```python
from build123d import *

# Parameters (mm, degrees)
SKETCH1_W           = 30
SKETCH1_H           = 60
SKETCH1_R           = 2
BOSS_EXTRUDE1_DEPTH = 3
SKETCH2_W           = 24
SKETCH2_H           = 3
BOSS_EXTRUDE2_DEPTH = 15
SKETCH3_R           = 2
CUT_EXTRUDE1_DEPTH  = 65.830548355
BOSS_EXTRUDE3_DEPTH = 2
SKETCH4_R           = 2.8
CUT_EXTRUDE2_DEPTH  = 2


with BuildPart() as part:
    # Sketch1 → Boss-Extrude1 (new body)
    with BuildSketch(Plane.XY):
        Rectangle(SKETCH1_W, SKETCH1_H)
        with Locations((8, 20)):
            Circle(SKETCH1_R, mode=Mode.SUBTRACT)
        with Locations(Location((8, -20, 0), (0, 0, 180))):
            Circle(SKETCH1_R, mode=Mode.SUBTRACT)
        with Locations(Location((-8, 20, 0), (0, 0, 180))):
            Circle(SKETCH1_R, mode=Mode.SUBTRACT)
        with Locations((-8, -20)):
            Circle(SKETCH1_R, mode=Mode.SUBTRACT)
    extrude(amount=BOSS_EXTRUDE1_DEPTH)

    # Sketch2 → Boss-Extrude2 (add, symmetric)
    with BuildSketch(Plane(origin=(0, 0, 0), x_dir=(0, 0, -1), z_dir=(1, 0, 0))):
        with Locations((-15, -28.5)):
            Rectangle(SKETCH2_W, SKETCH2_H)
    extrude(amount=BOSS_EXTRUDE2_DEPTH, both=True)

    # Sketch3 → Cut-Extrude1 (cut, through all)
    with BuildSketch(Plane(origin=(0, -27, 0), x_dir=(1, 0, 0), z_dir=(0, 1, 0))):
        with Locations(Location((-8, -6, 0), (0, 0, 270))):
            Circle(SKETCH3_R)
        with Locations(Location((8, -6, 0), (0, 0, 270))):
            Circle(SKETCH3_R)
        with Locations(Location((-8, -21, 0), (0, 0, 270))):
            Circle(SKETCH3_R)
        with Locations(Location((8, -21, 0), (0, 0, 270))):
            Circle(SKETCH3_R)
    extrude(amount=-CUT_EXTRUDE1_DEPTH, mode=Mode.SUBTRACT)

    # Sketch6 → Boss-Extrude3 (add, symmetric)
    with BuildSketch(Plane(origin=(0, 0, 0), x_dir=(0, 0, -1), z_dir=(1, 0, 0))):
        Polygon((-3, 30), (-27, -27), (-3, -27), align=None)
    extrude(amount=BOSS_EXTRUDE3_DEPTH, both=True)

    # Sketch4 → Cut-Extrude2 (cut)
    with BuildSketch(Plane(origin=(0, -27, 0), x_dir=(1, 0, 0), z_dir=(0, 1, 0))):
        with Locations(Location((-8, -6, 0), (0, 0, 270))):
            Circle(SKETCH4_R)
        with Locations(Location((8, -6, 0), (0, 0, 270))):
            Circle(SKETCH4_R)
    extrude(amount=-CUT_EXTRUDE2_DEPTH, mode=Mode.SUBTRACT)


solid = part.part
```
Part model, mm, in its own coordinate system. A direction names the side the tool comes from. Round coordinates to 2 decimals unless told otherwise and drop trailing zeros. Order: outer loops, then holes, each group sorted by start corner. A loop starts at its lowest first (then second) coordinate and runs counter-clockwise, first axis right, second up. Notation, with made-up numbers: M 33,18.25 L 72,18.25 A25 cw 72,42.25 Z; hole C -5,9 d2. An arc over 180 degrees is marked long. Put each result on its own line as item: value. Start each with the question number.
1. Drill centre lines: probe 1 along Y at (x, z) = (-8, 1.35); probe 2 along X at (y, z) = (-27.35, 6); probe 3 along Z at (x, y) = (-7.5, -9.5). Where is each one in solid material? Low to high. Write a range as [from, to].
2. Tool access for faces 5 (the face through (-6, -29, 5)), 6 (the face through (-8, -27, 15)), 7 (the face through (9, -27, 15)): list every direction of +Z, -Z, +X, -X, +Y, -Y with a clear straight run to the whole face (end or side of a thin tool).
3. Two-plate mould, pull along Z, no slides. Class faces 1 (the face through (2, -11, 10)), 2 (the face through (5.267, -27.986, 5.393)), 3 (the face through (0, 0, 0)), 4 (the face through (9.352, -28.479, 19.526)): +Z half, -Z half, draft (parallel to the pull), parting line (faces both ways), or undercut.
4. Drop flat-ended pins along their axis: pin 1 (6.5 mm diameter, centred on x = 7.5, y = 12, fed in from +Z); pin 2 (8 mm diameter, centred on y = -0.5, z = 19, fed in from -X); pin 3 (4 mm diameter, centred on x = 5.5, z = 13, fed in from +Y); pin 4 (3 mm diameter, centred on x = -8, z = 6, fed in from -Y). Give the stop position or say it passes through.
5. Slice it at C-C on y = -20. List the corners of the cut face in (x, z).
6. Slice it at A-A on x = -8. List the corners of the cut face in (y, z).
7. Slice it at B-B on z = 5.5. List the corners of the cut face in (x, y) (1 decimal), then the cut area to 3 significant figures.
8. Slice it at D-D on x = -12.75. List the corners of the cut face in (y, z), then the cut area to 3 significant figures.
Findings:
1. probe 1: [-30, -22], [-18, 18], [22, 30]
1. probe 2: [-15, -10.8], [-5.2, 5.2], [10.8, 15]
1. probe 3: [0, 3]
2. face 5: +Y
2. face 6: +Z, -X, +Y
2. face 7: +Z, +X, +Y
3. face 1: draft
3. face 2: undercut
3. face 3: -Z half
3. face 4: undercut
4. pin 1: z = 3
4. pin 2: x = -2
4. pin 3: y = -27
4. pin 4: through
5. outline: M -15,0 L -10,0 L -10,3 L -15,3 Z; M -6,0 L 6,0 L 6,3 L 2,3 L 2,24.05 L -2,24.05 L -2,3 L -6,3 Z; M 10,0 L 15,0 L 15,3 L 10,3 Z
6. outline: M -30,0 L -22,0 L -22,3 L -27,3 L -27,3.2 L -29,3.2 L -29,4 L -30,4 Z; M -30,8 L -29,8 L -29,8.8 L -27,8.8 L -27,19 L -30,19 Z; M -30,23 L -27,23 L -27,27 L -30,27 Z; M -18,0 L 18,0 L 18,3 L -18,3 Z; M 22,0 L 30,0 L 30,3 L 22,3 Z
7. outline: M -15,-30 L -9.9,-30 L -9.9,-29 L -10.8,-29 L -10.8,-27 L -15,-27 Z; M -6.1,-30 L 6.1,-30 L 6.1,-29 L 5.2,-29 L 5.2,-27 L 2,-27 L 2,24.1 L -2,24.1 L -2,-27 L -5.2,-27 L -5.2,-29 L -6.1,-29 Z; M 9.9,-30 L 15,-30 L 15,-27 L 10.8,-27 L 10.8,-29 L 9.9,-29 Z
7. area: 264 mm2
8. outline: M -30,0 L 30,0 L 30,3 L -27,3 L -27,27 L -30,27 Z
8. area: 252 mm2
